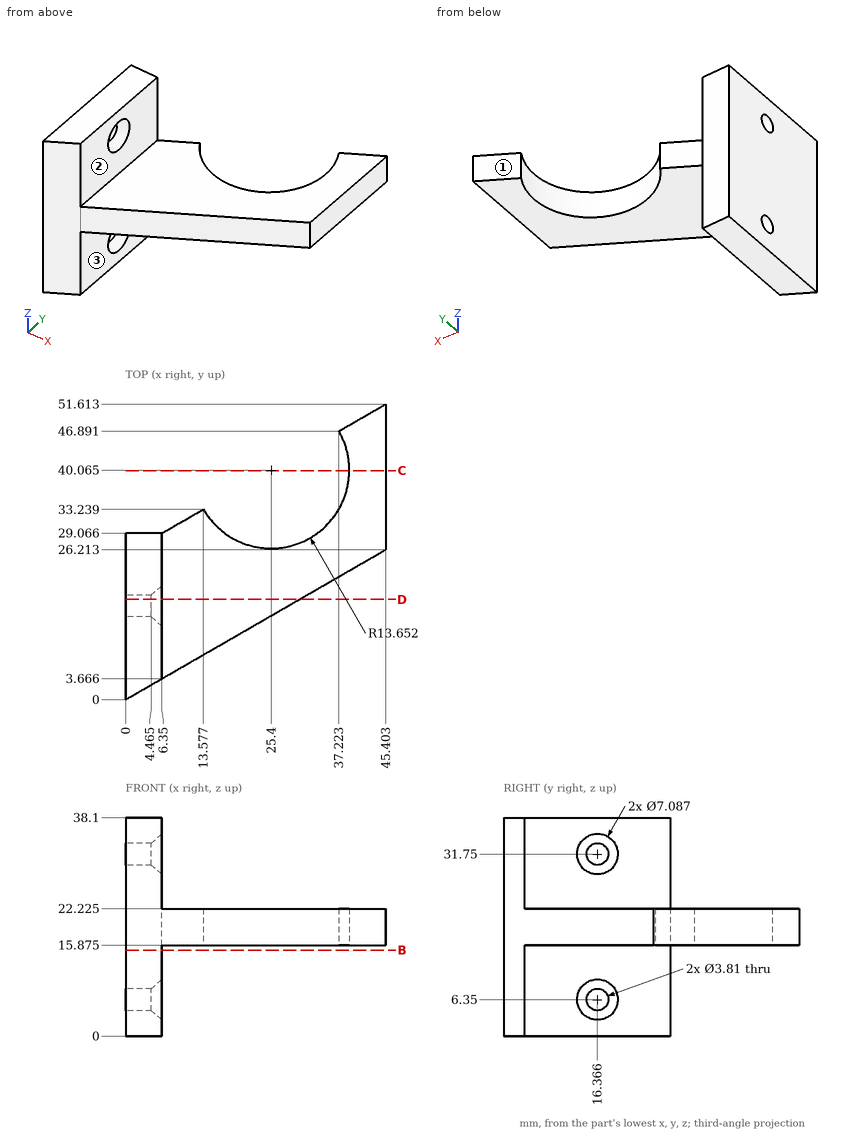
Part print with two shaded views. Sizes in mm from the minimum x, y, z corner. A direction names the side the tool comes from. Round coordinates to 2 decimals unless told otherwise and drop trailing zeros. Order: outer loops, then holes, each group sorted by start corner. A loop starts at its lowest first (then second) coordinate and runs counter-clockwise, first axis right, second up. Notation, with made-up numbers: M 42,31 L 78,31 A18 ccw 78,46 Z; hole C 16.5,35.25 d3. An arc over 180 degrees is marked long. Answer in a Markdown table with one row per item. Add a question column.
Q1. Pin check, flat tips, straight feed: pin 1 (11.5 mm diameter, centred on x = 33, y = 20.5, fed in from +Z) (1 decimal); pin 2 (12 mm diameter, centred on y = 30.5, z = 15.5, fed in from +X); pin 3 (2 mm diameter, centred on y = 36.5, z = 17, fed in from -X); pin 4 (8 mm diameter, centred on y = 13.5, z = 4, fed in from +X). Stop position of each tip, or through.
Q2. Cut at C-C on y = 40. Give the cut face in (x, z) (1 decimal), and give its area (3 significant figures).
Q3. Cut at D-D on y = 17.5. Give the number of separate pieces and of enclosed holes in the cut face, and give its area (3 significant figures).
Q4. Cut at B-B on z = 15. Give the cut face in (x, y).
Q5. Wall check: L1, parallel to X at y = 14.5, z = 27.5; L2, parallel to Y at x = 2.05, z = 31.75 (1 decimal); L3, parallel to Y at x = 2.9, z = 6.35 (1 decimal). Give the ranges that are in metal, low to high. Write a range as from..to.
Q6. 3-axis set-ups, long thin cutter, end or side, ignore diameter. For the marked faces 1, 2 and 3: which of +Z, -Z, +X, -X, +Y, -Y reach the whole face in a straight line?
Established:
| question | item | result |
|---|---|---|
| 1 | pin 1 | stops at z = 22.2 |
| 1 | pin 2 | stops at x = 45.4 |
| 1 | pin 3 | stops at x = 38.27 |
| 1 | pin 4 | stops at x = 6.35 |
| 2 | outline | M 39.1,15.9 L 45.4,15.9 L 45.4,22.2 L 39.1,22.2 Z |
| 2 | area | 40.3 mm2 |
| 3 | separate pieces | 3 |
| 3 | enclosed holes | 0 |
| 3 | area | 348 mm2 |
| 4 | outline | M 0,0 L 6.35,3.67 L 6.35,29.07 L 0,29.07 Z |
| 5 | L1 | x = 0..6.35 |
| 5 | L2 | y = 1.2..14.5, 18.3..29.1 |
| 5 | L3 | y = 1.7..14.5, 18.3..29.1 |
| 6 | face 1 | +Z, -Z, -X, +Y |
| 6 | face 2 | +Z, +X, +Y, -Y |
| 6 | face 3 | -Z, +X, +Y, -Y |
